from build123d import *

# Parameters (mm, degrees)
ESQUISSE1_W                  = 18
ESQUISSE1_H                  = 29
BOSS_EXTRU_1_DEPTH           = 46.2
ESQUISSE3_R                  = 1
ENL_V_MAT_EXTRU_1_DEPTH      = 58.440752084
ESQUISSE4_W                  = 18
ESQUISSE4_H                  = 30
ENL_V_MAT_EXTRU_2_DEPTH      = 58.440752084
ESQUISSE5_W                  = 8.1
ESQUISSE5_H                  = 46.2
BOSS_EXTRU_2_DEPTH           = 29
CONG_1_R                     = 3.5
ENL_V_START                  = -46.2
ESQUISSE7_W                  = 18
ESQUISSE7_H                  = 18
ENL_V_MAT_EXTRU_4_DEPTH      = 46.2
ESQUISSE8_W                  = 15
ESQUISSE8_H                  = 46.2
ESQUISSE8_R                  = 2.25
BOSS_EXTRU_3_DEPTH           = 11
CHANFREIN1_SIZE              = 9
CONG_2_R                     = 3.5
ENL_V_MAT_EXTRU_5_DEPTH      = 65.402251513
ENL_V_MAT_EXTRU_5_DEPTH_BACK = 65.402251513
ESQUISSE9_W                  = 25.1
ESQUISSE9_H                  = 38.1
CHANFREIN2_SIZE              = 16


with BuildPart() as part:
    # Esquisse1 → Boss.-Extru.1 (new body)
    with BuildSketch(Plane.XY):
        with Locations((9, 14.5)):
            Rectangle(ESQUISSE1_W, ESQUISSE1_H)
    extrude(amount=BOSS_EXTRU_1_DEPTH)

    # Esquisse3 → Enl_v. mat.-Extru.1 (cut, through all)
    with BuildSketch(Plane.XY.offset(46.2)):
        with Locations((2.5, 26.2)):
            Circle(ESQUISSE3_R)
        with Locations((2.5, 9.2)):
            Circle(ESQUISSE3_R)
    extrude(amount=-ENL_V_MAT_EXTRU_1_DEPTH, mode=Mode.SUBTRACT)

    # Esquisse4 → Enl_v. mat.-Extru.2 (cut, through all)
    with BuildSketch(Plane(origin=(0, 29, 0), x_dir=(1, 0, 0), z_dir=(0, 1, 0))):
        with Locations((9, -23.1)):
            Rectangle(ESQUISSE4_W, ESQUISSE4_H)
    extrude(amount=-ENL_V_MAT_EXTRU_2_DEPTH, mode=Mode.SUBTRACT)


with BuildPart() as enl_v_mat_extru_2_piece_1:
    # of the separate pieces the step leaves, piece 1, a body of its own (enl_v_mat_extru_2_pieces)
    add(part.part.solids().sort_by_distance((0, 0, 0))[0])



with BuildPart() as enl_v_mat_extru_2_piece_2:
    # of the separate pieces the step leaves, piece 2, a body of its own (enl_v_mat_extru_2_pieces)
    add(part.part.solids().sort_by_distance((18, 0, 38.1))[0])


with BuildPart() as enl_v_mat_extru_2_piece_1_1:
    add(enl_v_mat_extru_2_piece_1.part)

    add(enl_v_mat_extru_2_piece_2.part)  # Boss.-Extru.2 merges Enl_v. mat.-Extru.2 piece 2
    # Esquisse5 → Boss.-Extru.2 (add)
    with BuildSketch(Plane(origin=(0, 29, 0), x_dir=(1, 0, 0), z_dir=(0, 1, 0))):
        with Locations((22.05, -23.1)):
            Rectangle(ESQUISSE5_W, ESQUISSE5_H)
    extrude(amount=-BOSS_EXTRU_2_DEPTH)

    # Cong_1
    cong_1_edges = [enl_v_mat_extru_2_piece_1_1.edges().sort_by_distance(p)[0] for p in [
        (0, 29, 42.15),
        (0, 29, 4.05),
    ]]
    fillet(cong_1_edges, radius=CONG_1_R)

    # Esquisse7 → Enl_v. mat.-Extru.4 (cut)
    with BuildSketch(Plane(origin=(0, 0, 0), x_dir=(-1, 0, 0), z_dir=(0, 0, -1)).offset(ENL_V_START)):
        with Locations((-17.1, 20)):
            Rectangle(ESQUISSE7_W, ESQUISSE7_H)
    extrude(amount=ENL_V_MAT_EXTRU_4_DEPTH, mode=Mode.SUBTRACT)

    # Esquisse8 → Boss.-Extru.3 (add)
    with BuildSketch(Plane(origin=(0, 11, 0), x_dir=(1, 0, 0), z_dir=(0, 1, 0))):
        with Locations((33.6, -23.1)):
            Rectangle(ESQUISSE8_W, ESQUISSE8_H)
        with Locations(Location((33.6, -5.5, 0), (0, 0, 270))):
            Circle(ESQUISSE8_R, mode=Mode.SUBTRACT)
        with Locations(Location((33.6, -32.5, 0), (0, 0, 270))):
            Circle(ESQUISSE8_R, mode=Mode.SUBTRACT)
        with Locations(Location((33.6, -19, 0), (0, 0, 270))):
            Circle(ESQUISSE8_R, mode=Mode.SUBTRACT)
    extrude(amount=-BOSS_EXTRU_3_DEPTH)

    # Chanfrein1
    chanfrein1_edges = [enl_v_mat_extru_2_piece_1_1.edges().sort_by_distance(p)[0] for p in [
        (8.1, 11, 42.15),
        (8.1, 11, 4.05),
    ]]
    chamfer(chanfrein1_edges, length=CHANFREIN1_SIZE)

    # Cong_2
    cong_2_edges = [enl_v_mat_extru_2_piece_1_1.edges().sort_by_distance(p)[0] for p in [
        (8.1, 29, 42.15),
        (8.1, 29, 4.05),
    ]]
    fillet(cong_2_edges, radius=CONG_2_R)

    # Esquisse9 → Enl_v. mat.-Extru.5 (cut, two sides: drawn at the far end of the back side and taken through both)
    with BuildSketch(Plane(origin=(0, 11, 0), x_dir=(1, 0, 0), z_dir=(0, 1, 0)).offset(-ENL_V_MAT_EXTRU_5_DEPTH_BACK)):
        with Locations((12.55, -27.15)):
            Rectangle(ESQUISSE9_W, ESQUISSE9_H)
    extrude(amount=ENL_V_MAT_EXTRU_5_DEPTH + ENL_V_MAT_EXTRU_5_DEPTH_BACK, mode=Mode.SUBTRACT)

    # Chanfrein2
    chanfrein2_edges = [enl_v_mat_extru_2_piece_1_1.edges().sort_by_distance(p)[0] for p in [
        (25.1, 5.5, 8.1),
    ]]
    chamfer(chanfrein2_edges, length=CHANFREIN2_SIZE)


solid = enl_v_mat_extru_2_piece_1_1.part
The listing builds one solid part. Answer for the finished solid, in the listing's coordinates (mm). A direction names the side the tool comes from. Round coordinates to 2 decimals unless told otherwise and drop trailing zeros. Order: outer loops, then holes, each group sorted by start corner. A loop starts at its lowest first (then second) coordinate and runs counter-clockwise, first axis right, second up. Notation, with made-up numbers: M 19.25,67.5 L 51.25,67.5 A23 ccw 51.25,88.5 Z; hole C -33,74 d8. An arc over 180 degrees is marked long. Answer in a Markdown table with one row per item. Add a question column.
1) The part is cut by section C-C on y = 4.75. Determine the outline of the cut face in (x, z), plus the area to 3 significant figures.
2) The part is cut by section B-B on z = 19. Determine the outline of the cut face in (x, y).
3) Determine the mould class of faces 1 (the face through (33, 6, 46.2)), 2 (the face through (35.497, 5.577, 6.71)), 3 (the face through (0, 13, 4)) for opening direction Z: pulls with the +Z half, pulls with the -Z half, needs draft (parallel to the pull), parting line crosses it, or undercut.
4) Consider line 1 along X through (y, z) = (4.75, 32.5); line 2 along X through (y, z) = (7, 10); line 3 along Y through (x, z) = (2, 3). Determine where each line is inside the solid, lowest interval first. Write a range as from..to.
5) The part is cut by section A-A on z = 5.5. Determine the outline of the cut face in (x, y), plus the area to 3 significant figures.
6) The part is cut by section D-D on x = 34.5. Determine the outline of the cut face in (y, z), plus the area to 3 significant figures.
7) Which of the six approach directions +Z, -Z, +X, -X, +Y, -Y give full straight-line access (tool end or side, diameter ignored) to faces 4 (the face through (1, 27.95, 4.11)), 5 (the face through (4, 14, 8.1)), 6 (the face through (32, 11, 23))?
8) Flat-ended cylindrical pins translate along their axes: pin 1 Ø9 at (y, z) = (7.5, 38.5) entering from -X; pin 2 Ø6 at (y, z) = (24, 10.5) entering from +X; pin 3 Ø19 at (x, z) = (32.5, 17) entering from +Y. Find the tip coordinate at first contact, or state that the pin passes through.
Findings below:
| question | item | result |
|---|---|---|
| 1 | outline | M 0,0 L 41.1,0 L 41.1,46.2 L 25.1,46.2 L 25.1,24.1 L 9.1,8.1 L 0,8.1 Z; hole C 33.6,5.5 d4.5; hole C 33.6,19 d4.5; hole C 33.6,32.5 d4.5 |
| 1 | area | 1,020 mm² |
| 2 | outline | M 20,0 L 31.35,0 L 31.35,11 L 20,11 Z; M 35.85,0 L 41.1,0 L 41.1,11 L 35.85,11 Z |
| 3 | face 1 | pulls with the +Z half |
| 3 | face 2 | undercut |
| 3 | face 3 | needs draft |
| 4 | line 1 | x = 25.1..31.35, 35.85..41.1 |
| 4 | line 2 | x = 11..41.1 |
| 4 | line 3 | y = 0..8.33, 10.07..25.33, 27.07..28.66 |
| 5 | outline | M 0,0 L 31.35,0 L 31.35,11 L 17.1,11 L 8.1,20 L 8.1,25.5 A3.5 ccw 4.6,29 L 3.5,29 A3.5 ccw 0,25.5 Z; M 35.85,0 L 41.1,0 L 41.1,11 L 35.85,11 Z; hole C 2.5,9.2 d2; hole C 2.5,26.2 d2 |
| 5 | area | 577 mm² |
| 6 | outline | M 0,0 L 11,0 L 11,3.44 L 0,3.44 Z; M 0,7.56 L 11,7.56 L 11,16.94 L 0,16.94 Z; M 0,21.06 L 11,21.06 L 11,30.44 L 0,30.44 Z; M 0,34.56 L 11,34.56 L 11,46.2 L 0,46.2 Z |
| 6 | area | 372 mm² |
| 7 | face 4 | +Z, -Z, -X, +Y |
| 7 | face 5 | +Z, -X, +Y, -Y |
| 7 | face 6 | +Z, -Z, +X, +Y |
| 8 | pin 1 | stops at x = 25.1 |
| 8 | pin 2 | stops at x = 8.1 |
| 8 | pin 3 | stops at y = 11 |
